from build123d import *

# Parameters (mm, degrees)
SKETCH1_R           = 18.5
BOSS_EXTRUDE1_DEPTH = 29
CUT_EXTRUDE1_START  = -31.5
SKETCH2_R           = 18.5
SKETCH2_R_2         = 17.25
CUT_EXTRUDE1_DEPTH  = 31.5
SKETCH3_R           = 6
BOSS_EXTRUDE2_DEPTH = 6
SKETCH4_R           = 3
BOSS_EXTRUDE3_DEPTH = 15
CUT_EXTRUDE2_START  = -12
CUT_EXTRUDE2_DEPTH  = 12
CIRPATTERN1_COUNT   = 6


with BuildPart() as part:
    # Sketch1 → Boss-Extrude1 (new, symmetric)
    with BuildSketch(Plane.XY):
        with Locations(Location((0, 0, 0), (0, 0, 180))):
            Circle(SKETCH1_R)
    extrude(amount=BOSS_EXTRUDE1_DEPTH, both=True)

    # Sketch2 → Cut-Extrude1 (cut)
    with BuildSketch(Plane(origin=(0, 0, -29), x_dir=(-1, 0, 0), z_dir=(0, 0, -1)).offset(CUT_EXTRUDE1_START)):
        Circle(SKETCH2_R)
        Circle(SKETCH2_R_2, mode=Mode.SUBTRACT)
    extrude(amount=CUT_EXTRUDE1_DEPTH, mode=Mode.SUBTRACT)

    # Sketch3 → Boss-Extrude2 (add)
    with BuildSketch(Plane.XY.offset(29)):
        with Locations((0, 7)):
            Circle(SKETCH3_R)
    extrude(amount=BOSS_EXTRUDE2_DEPTH)

    # Sketch4 → Boss-Extrude3 (add)
    with BuildSketch(Plane.XY.offset(35)):
        with Locations((0, 7)):
            Circle(SKETCH4_R)
    extrude(amount=BOSS_EXTRUDE3_DEPTH)

    # Sketch5 → Cut-Extrude2 (cut)
    with BuildSketch(Plane.XY.offset(50).offset(CUT_EXTRUDE2_START)):
        with BuildLine():
            Line((-1.658312395, 9.5), (1.658312395, 9.5))
            ThreePointArc((1.658312395, 9.5), (0, 10), (-1.658312395, 9.5))
        make_face()
    extrude(amount=CUT_EXTRUDE2_DEPTH, mode=Mode.SUBTRACT)

    # Sketch7 → M3x0.5 Tapped Hole1 (revolve, cut)
    with BuildSketch(Plane(origin=(7.75, 13.423393759, 29), x_dir=(0, -1, 0), z_dir=(1, 0, 0))):
        Polygon((0, 0), (0, 4.251075774), (1.25, 3.5), (1.25, 0), align=None)
    m3x0_5_tapped_hole1 = revolve(axis=Axis((7.75, 13.423393759, 35.35), (0, 0, -1)), mode=Mode.SUBTRACT)

    # CirPattern1: M3x0.5 Tapped Hole1 ×6 about axis
    cirpattern1_axis = Axis((0, 0, 0), (0, 0, 1))
    for i in range(1, CIRPATTERN1_COUNT):
        add(m3x0_5_tapped_hole1.rotate(cirpattern1_axis, i * 360 / CIRPATTERN1_COUNT), mode=Mode.SUBTRACT)


solid = part.part
Can you work these out from the model? Positions are in its coordinate system, mm. A direction names the side the tool comes from. Coordinates: 2 decimals unless noted, no trailing zeros. Write each loop counter-clockwise with the first axis right and the second up, starting at its lowest first coordinate (ties: lowest second). Pieces come first, ordered by that corner, then holes. Notation, with made-up numbers: (80, -17.75) -> (136, -17.75) arc R12 cw to (136, 0.25) -> close; hole circle Ø8 at (38, 18.5). An arc over 180 degrees is marked (long way). Answer as CSV lines item,"result".
1) Will these pins go through, and if not, where does the flat tip stop? P1, Ø2, axis at x = 0, z = -8, coming from the -Y side; P2, Ø2.5, axis at x = -0.5, z = 46, coming from the +Y side; P3, Ø1.5, axis at x = -7.75, y = 13.42, coming from the +Z side.
Check result:
P1,"y = -17.25"
P2,"y = 9.5"
P3,"z = 25.2"
2) If we section it at A-A on y = 7: Please give me the cut outline in (x, z), then the cut area to 3 significant figures.
Check result:
outline,"(-17.12, 2.5) -> (-15.77, 2.5) -> (-15.77, -29) -> (15.77, -29) -> (15.77, 2.5) -> (17.12, 2.5) -> (17.12, 29) -> (6, 29) -> (6, 35) -> (3, 35) -> (3, 50) -> (-3, 50) -> (-3, 35) -> (-6, 35) -> (-6, 29) -> (-17.12, 29) -> close"
area,"2,060 mm²"
3) If I drill on line 1 (X direction, y = 0, z = 28.35); line 2 (Y direction, x = 7, z = 27); line 3 (Z direction, x = 8.5, y = 6), over which ranges is the centre line in solid material (lowest first)? Write a range as from..to.
Check result:
line 1,"-18.5..-16.75, -14.25..14.25, 16.75..18.5"
line 2,"-17.12..-14.42, -12.42..12.42, 14.42..17.12"
line 3,"-29..29"
4) If we section it at D-D on y = -8: Please give me the cut outline in (x, z).
Check result:
outline,"(-16.68, 2.5) -> (-15.28, 2.5) -> (-15.28, -29) -> (15.28, -29) -> (15.28, 2.5) -> (16.68, 2.5) -> (16.68, 29) -> (-16.68, 29) -> close"
5) If we mould it in two halves opening along X, with no side actions, what happens to faces 4 (the cylindrical face through (-16.453, 5.181, -13.03)), 5 (the flat face through (17, -5, 2.5)), 6 (the cylindrical face through (-8.86, 14, 27.27))? For each: +X half, -X half, draft (parallel to the pull), parting line (faces both ways), or undercut.
Check result:
face 4,"parting line"
face 5,"draft"
face 6,"undercut"
6) On a 3-axis mill with a long thin cutter (end or side, diameter ignored), from which of +Z, -Z, +X, -X, +Y, -Y can I reach the whole of each face in a straight line? I mean faces 1 (the cylindrical face through (8.86, -14, 27.27)), 2 (the flat face through (0, 9.5, 44)), 3 (the flat face through (0, 7, 50)). Say none if no direction works.
Check result:
face 1,"+Z"
face 2,"+Z, +X, -X, +Y"
face 3,"+Z, +X, -X, +Y, -Y"
7) If we section it at C-C on z = 14: Please give me the cut outline in (x, y).
Check result:
outline,"circle Ø37 at (0, 0)"
8) If we section it at B-B on x = -5: Please give me the cut outline in (y, z), then the cut area to 3 significant figures.
Check result:
outline,"(-17.81, 2.5) -> (-16.51, 2.5) -> (-16.51, -29) -> (16.51, -29) -> (16.51, 2.5) -> (17.81, 2.5) -> (17.81, 29) -> (10.32, 29) -> (10.32, 35) -> (3.68, 35) -> (3.68, 29) -> (-17.81, 29) -> close"
area,"2,020 mm²"
